```python
from build123d import *

# Parameters (mm, degrees)
ESBO_O1_R                = 1.5
ESBO_O1_W                = 3
ESBO_O1_H                = 8
ESBO_O1_W_2              = 8
ESBO_O1_H_2              = 3
RESSALTO_EXTRUS_O1_DEPTH = 3


with BuildPart() as part:
    # Esboço1 → Ressalto-extrusão1 (new body)
    with BuildSketch(Plane(origin=(0, 0, 0), x_dir=(1, 0, 0), z_dir=(0, 1, 0))):
        with BuildLine():
            Line((-4.674449837, 5.126823449), (2.15649844, 5.74992269))
            add(Edge.make_bspline(
                [(19.127700004, 3.859391667), (13.692888976, 5.757269931), (8.035822873, 6.387450044), (2.15649844, 5.74992269)],
                knots=[0.35388944, 0.35388944, 0.35388944, 0.35388944, 1, 1, 1, 1], degree=3))
            ThreePointArc((19.127700004, 3.859391667), (21.595587829, 3.06871935), (24.101127023, 2.406974398))
            add(Edge.make_bspline(
                [(24.101129521, -3.20712694), (35.966754752, -0.40007519), (24.101127023, 2.406974398)],
                knots=[5.194112275, 5.194112275, 5.194112275, 7.372258742, 7.372258742, 7.372258742], degree=2, weights=[1, 0.463306864, 1]))
            ThreePointArc((24.101129521, -3.20712694), (21.595589041, -3.868872862), (19.127700004, -4.659546287))
            add(Edge.make_bspline(
                [(19.127700004, -4.659546287), (13.692889505, -6.55742607), (8.035822337, -7.187603127), (2.15649844, -6.55007731)],
                knots=[0.35388944, 0.35388944, 0.35388944, 0.35388944, 1, 1, 1, 1], degree=3))
            Line((2.15649844, -6.55007731), (-4.674449837, -5.926978069))
            add(Edge.make_bspline(
                [(-23.759026807, -13.92609603), (-18.993134449, -8.145749128), (-12.424143506, -5.367564321), (-4.674449837, -5.926978069)],
                knots=[0.101821695, 0.101821695, 0.101821695, 0.101821695, 1, 1, 1, 1], degree=3))
            ThreePointArc((-23.759026807, -13.92609603), (-25.800414194, -15.798822034), (-28.277263571, -17.039621097))
            add(Edge.make_bspline(
                [(-28.277263571, -17.039621097), (-34.579205058, -19.166234), (-47.597806191, -22.747709276), (-59.650258973, -23.294853785), (-64.986052109, -22.387135922)],
                knots=[0.241589655, 0.241589655, 0.241589655, 0.241589655, 0.401358205, 0.561126756, 0.561126756, 0.561126756, 0.561126756], degree=3))
            ThreePointArc((-64.986052109, -22.387135922), (-69.209775007, -20.602207926), (-72.192804257, -17.119774932))
            ThreePointArc((-72.192804257, -17.119774932), (-76.257665323, -0.40007754), (-72.192804468, 16.319619904))
            ThreePointArc((-72.192804468, 16.319619904), (-69.209774999, 19.802053128), (-64.986051746, 21.586981094))
            add(Edge.make_bspline(
                [(-28.2772637, 16.239466453), (-34.57920511, 18.366079177), (-47.597806077, 21.947554059), (-59.650258689, 22.494698656), (-64.986051746, 21.586981094)],
                knots=[0.241589656, 0.241589656, 0.241589656, 0.241589656, 0.401358204, 0.561126752, 0.561126752, 0.561126752, 0.561126752], degree=3))
            ThreePointArc((-28.2772637, 16.239466453), (-25.80041422, 14.998667392), (-23.759026751, 13.125941342))
            add(Edge.make_bspline(
                [(-23.759026751, 13.125941342), (-18.993134399, 7.345594488), (-12.424143468, 4.567409699), (-4.674449837, 5.126823449)],
                knots=[0.101821698, 0.101821698, 0.101821698, 0.101821698, 1, 1, 1, 1], degree=3))
        make_face()
        with Locations((-45.242023738, 13.89992269)):
            Circle(ESBO_O1_R, mode=Mode.SUBTRACT)
        with Locations((-68.242023738, -14.70007731)):
            Circle(ESBO_O1_R, mode=Mode.SUBTRACT)
        with Locations((-59.742023738, 11.09992269)):
            Circle(ESBO_O1_R, mode=Mode.SUBTRACT)
        with Locations((-31.142023738, -11.40175485)):
            Circle(ESBO_O1_R, mode=Mode.SUBTRACT)
        with Locations((-39.142023738, -0.40007731)):
            Circle(ESBO_O1_R, mode=Mode.SUBTRACT)
        with Locations((10.857976262, -0.40007731)):
            Circle(ESBO_O1_R, mode=Mode.SUBTRACT)
        with Locations((-1.642023738, -0.40007731)):
            Circle(ESBO_O1_R, mode=Mode.SUBTRACT)
        with Locations((-26.642023738, -0.40007731)):
            Circle(ESBO_O1_R, mode=Mode.SUBTRACT)
        with Locations((-45.242023738, -14.70007731)):
            Rectangle(ESBO_O1_W, ESBO_O1_H, mode=Mode.SUBTRACT)
        with Locations((-68.242023738, 13.89992269)):
            Rectangle(ESBO_O1_W, ESBO_O1_H, mode=Mode.SUBTRACT)
        with Locations((-31.142023738, 11.099922699)):
            Rectangle(ESBO_O1_W_2, ESBO_O1_H_2, mode=Mode.SUBTRACT)
        with Locations((-59.742023738, -11.90007731)):
            Rectangle(ESBO_O1_W_2, ESBO_O1_H_2, mode=Mode.SUBTRACT)
    extrude(amount=RESSALTO_EXTRUS_O1_DEPTH)


solid = part.part
```
Geometry: final body of the model. Coordinates: model frame, mm. A direction names the side the tool comes from. Round coordinates to 2 decimals unless told otherwise and drop trailing zeros. Answer in a Markdown table with one row per item. Add a question column.
(1) Ray query, L1, parallel to X at y = 2.6, z = 15.5; L2, parallel to Z at x = -30.5, y = 1; L3, parallel to X at y = 1.05, z = 14. Return the intervals inside material, ascending.
(2) Contact query for flat-ended pins moving along their axis: pin 1 (0.9 mm diameter, centred on y = 1, z = 11, fed in from +X); pin 2 (0.9 mm diameter, centred on y = 1, z = 12.5, fed in from -X); pin 3 (0.9 mm diameter, centred on x = -60, y = 2, fed in from +Z). Output: stop coordinate, or through.
(3) Draft query along Z for faces 1 (the face through (-0.256, 1.479, 0.975)), 2 (the face through (-25.8, 1.5, 15.8)), 3 (the face through (-44, 3, 0)). Return one class per face: pulls with the +Z half, pulls with the -Z half, needs draft (parallel to the pull), parting line crosses it, or undercut.
(4) Cut plane A-A, the plane y = 1.35. Give the number of separate pieces and of enclosed holes in the cut face, then the cut area to 3 significant figures.
(5) Reachability of faces 4 (the face through (21.63, 1.48, 3.86)), 5 (the face through (-68, 1, -9.9)), 6 (the face through (-1.307, 1.479, -5.434)) from +Z, -Z, +X, -X, +Y, -Y: full face, straight path, thin tool, end or side. Return the list, or none.
Established:
| question | item | result |
|---|---|---|
| 1 | L1 | -72.98 to -69.51, -66.97 to -46.74, -43.74 to -25.39 |
| 1 | L2 | -16.97 to -12.6, -9.6 to 10.05, 12.76 to 17.77 |
| 1 | L3 | -73.62 to -69.57, -66.92 to -46.74, -43.74 to -23.82 |
| 2 | pin 1 | x = -20.36 |
| 2 | pin 2 | x = -74.34 |
| 2 | pin 3 | z = 22.91 |
| 3 | face 1 | undercut |
| 3 | face 2 | pulls with the +Z half |
| 3 | face 3 | needs draft |
| 4 | separate pieces | 1 |
| 4 | enclosed holes | 12 |
| 4 | area | 2,510 mm² |
| 5 | face 4 | +Z, +X, +Y, -Y |
| 5 | face 5 | +Y, -Y |
| 5 | face 6 | -Z, +Y, -Y |
